```python
from build123d import *

# Parameters (mm, degrees)
SKETCH_1_R      = 1.75
SKETCH_1_R_2    = 10
EXTRUDE_1_DEPTH = 3


with BuildPart() as part:
    # Эскиз1 → Бобышка-Вытянуть1 (new body)
    with BuildSketch(Plane.XY):
        with BuildLine():
            Line((29.589201296, 3.75), (18.042195912, 23.75))
            ThreePointArc((18.042195912, 23.75), (15.297005384, 26.495190528), (11.547005384, 27.5))
            Line((11.547005384, 27.5), (-11.547005384, 27.5))
            ThreePointArc((-11.547005384, 27.5), (-15.297005384, 26.495190528), (-18.042195912, 23.75))
            Line((-18.042195912, 23.75), (-29.589201296, 3.75))
            ThreePointArc((-29.589201296, 3.75), (-30.594010768, 0), (-29.589201296, -3.75))
            Line((-29.589201296, -3.75), (-18.042195912, -23.75))
            ThreePointArc((-18.042195912, -23.75), (-15.297005384, -26.495190528), (-11.547005384, -27.5))
            Line((-11.547005384, -27.5), (11.547005384, -27.5))
            ThreePointArc((11.547005384, -27.5), (15.297005384, -26.495190528), (18.042195912, -23.75))
            Line((18.042195912, -23.75), (29.589201296, -3.75))
            ThreePointArc((29.589201296, -3.75), (30.594010768, 0), (29.589201296, 3.75))
        make_face()
        with Locations((0, 24)):
            Circle(SKETCH_1_R, mode=Mode.SUBTRACT)
        with Locations((20.784609691, -12)):
            Circle(SKETCH_1_R, mode=Mode.SUBTRACT)
        with Locations((-20.784609691, -12)):
            Circle(SKETCH_1_R, mode=Mode.SUBTRACT)
        Circle(SKETCH_1_R_2, mode=Mode.SUBTRACT)
    extrude(amount=EXTRUDE_1_DEPTH)


solid = part.part
```
Geometry: final body of the model. Coordinates: model frame, mm. Round coordinates to 2 decimals unless told otherwise and drop trailing zeros. Order: outer loops, then holes, each group sorted by start corner. A loop starts at its lowest first (then second) coordinate and runs counter-clockwise, first axis right, second up. Notation, with made-up numbers: (44.25, 36) - (86.25, 36) arc R27 cw to (86.25, 73) - close; hole circle Ø4 at (35.5, 42.5). An arc over 180 degrees is marked (long way). Use CSV: the item, a comma, the result in double quotes. Start each with the question number.
Q1. Section query A-A (x = 8). Return loops of the section in (y, z).
Q2. Material intervals for line 1 along Y through (x, z) = (0, 1.9); line 2 along Y through (x, z) = (-2.5, 1.8); line 3 along X through (y, z) = (22.5, 2.9), sorted ascending. Write a range as from..to.
Q3. First-contact query: pin 1 (2 mm diameter, centred on x = 12.5, y = 16.5, fed in from -Z); pin 2 (12 mm diameter, centred on x = 0, y = 0, fed in from -Z); pin 3 (1 mm diameter, centred on x = 21.5, z = 1.5, fed in from -Y). Flat tips, straight axial feed; report the tip coordinate or a pass-through.
Q4. Section query C-C (z = 1.3). Return loops of the section in (x, y).
Q5. Section query D-D (x = 0). Return loops of the section in (y, z).
Q6. Mould query, pull axis X, two halves, no side actions, for faces 1 (the face through (0, -27.5, 1)), 2 (the face through (-0.228, 25.735, 1.479)), 3 (the face through (-15.34, -26.47, 1.48)). Classes: +X half, -X half, draft (parallel to the pull), parting line (faces both ways), or undercut.
Q7. Section query B-B (y = 0). Return loops of the section in (x, z).
Result set:
1,outline,"(-27.5, 0) - (-6, 0) - (-6, 3) - (-27.5, 3) - close; (6, 0) - (27.5, 0) - (27.5, 3) - (6, 3) - close"
2,line 1,"y = -27.5..-10, 10..22.25, 25.75..27.5"
2,line 2,"y = -27.5..-9.68, 9.68..27.5"
2,line 3,"x = -18.76..-0.9, 0.9..18.76"
3,pin 1,"stops at z = 0"
3,pin 2,"passes through"
3,pin 3,"stops at y = -18.63"
4,outline,"(-29.59, -3.75) - (-18.04, -23.75) arc R7.5 ccw to (-11.55, -27.5) - (11.55, -27.5) arc R7.5 ccw to (18.04, -23.75) - (29.59, -3.75) arc R7.5 ccw to (29.59, 3.75) - (18.04, 23.75) arc R7.5 ccw to (11.55, 27.5) - (-11.55, 27.5) arc R7.5 ccw to (-18.04, 23.75) - (-29.59, 3.75) arc R7.5 ccw to start; hole circle Ø3.5 at (-20.78, -12); hole circle Ø20 at (0, 0); hole circle Ø3.5 at (0, 24); hole circle Ø3.5 at (20.78, -12)"
5,outline,"(-27.5, 0) - (-10, 0) - (-10, 3) - (-27.5, 3) - close; (10, 0) - (22.25, 0) - (22.25, 3) - (10, 3) - close; (25.75, 0) - (27.5, 0) - (27.5, 3) - (25.75, 3) - close"
6,face 1,"draft"
6,face 2,"undercut"
6,face 3,"-X half"
7,outline,"(-30.59, 0) - (-10, 0) - (-10, 3) - (-30.59, 3) - close; (10, 0) - (30.59, 0) - (30.59, 3) - (10, 3) - close"
